from build123d import *

# Parameters (mm, degrees)
F0_W      = 114.3
F0_H      = 60.325
F1_DEPTH  = 42.8625
F2_W      = 98.425
F2_H      = 31.75
F3_DEPTH  = 25.4
F4_R      = 7.9375
F5_DEPTH  = 25.4
F10_DEPTH = 127


with BuildPart() as f1:
    # F0 (on Front) → F1 (new body, symmetric)
    with BuildSketch(Plane.XZ):
        with Locations((57.15, 30.1625)):
            Rectangle(F0_W, F0_H)
    extrude(amount=F1_DEPTH, both=True)

    # F2 (on face) → F3 (join)
    with BuildSketch(Plane.XY.offset(60.325)):
        with Locations((65.0875, -12.7)):
            Rectangle(F2_W, F2_H)
    extrude(amount=F3_DEPTH)

    # F4 (on face) → F5 (cut)
    with BuildSketch(Plane.XY.offset(60.325)):
        with Locations((31.8531343792, -12.7)):
            Circle(F4_R)
    extrude(amount=F5_DEPTH, mode=Mode.SUBTRACT)

    # F9 (on 3pt) → F10 (cut)
    with BuildSketch(Plane(origin=(85.5876450588, -49.4525301974, 49.4525301974), x_dir=(0.3874037681, 0.8943227315, 0.2238418469), z_dir=(0.7743554069, -0.4474224535, 0.4474224535))):
        Polygon((-14.9042876437, -25.4722796381), (7.5109787285, -51.4674633741), (114.2435371876, -48.7483553588), (131.361335516, 53.0414171517), (24.5024245232, 35.0616015494), (7.6925121248, 10.4205505922), align=None)
    extrude(amount=F10_DEPTH, mode=Mode.SUBTRACT)


solid = f1.part
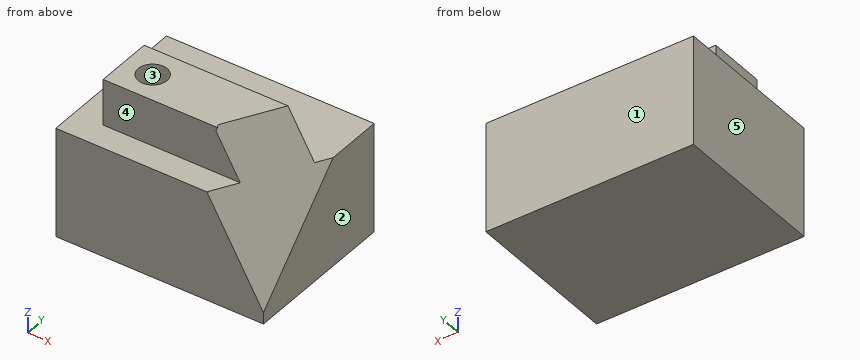
Work out the finished part from the listing and answer in its coordinate system (mm). Face numbers are marked on the shaded views. A direction names the side the tool comes from. Give positions to 0.01 mm unless a question says otherwise; leave off trailing zeros. Write each loop counter-clockwise with the first axis right and the second up, starting at its lowest first coordinate (ties: lowest second). Pieces come first, ordered by that corner, then holes. Notation, with made-up numbers: M 88.25,56 L 115.25,56 A19 ccw 115.25,70 Z; hole C 46,-23.75 d5. An arc over 180 degrees is marked long. Answer as CSV lines item,"result".
Q1. Given P1, Ø4, axis at x = 59.5, y = 14.5, coming from the +Z side (3 decimals); P2, Ø12.5, axis at x = 71.5, z = 74, coming from the -Y side (3 decimals); P3, Ø12.5, axis at x = 74, z = 68, coming from the +Y side (3 decimals), each flat-ended and moving along its own axis, determine where each tip first touches the part or whether it passes through.
A:
P1,"stops at z = 60.325"
P2,"stops at y = -28.575"
P3,"stops at y = 3.175"
Q2. A cutting plane is placed at C-C on z = 48. Write down the section's boundary in (x, y).
A:
outline,"M 0,-42.86 L 90.23,-42.86 L 114.3,-1.21 L 114.3,42.86 L 0,42.86 Z"
Q3. A tool of negligible diameter and unlimited length cuts with its end or side. For the marked faces 4 and 5, from which of +Z, -Z, +X, -X, +Y, -Y can it reach the whole face along a straight path? Write none if from no direction.
A:
face 4,"+Z, +X, -X, -Y"
face 5,"+Z, -Z, -X, +Y, -Y"
Q4. A cutting plane is placed at B-B on y = -1. Write down the section's boundary in (x, z) (1 decimal), plus the area to 3 significant figures.
A:
outline,"M 0,0 L 114.3,0 L 114.3,48.2 L 92.6,85.7 L 15.9,85.7 L 15.9,60.3 L 0,60.3 Z"
area,"8,990 mm²"
Q5. Find the intervals of material crossed by probe 1 along Z at (x, y) = (7.5, -11.5) (3 decimals); probe 2 along Y at (x, z) = (64.5, 66.5) (3 decimals); probe 3 along Y at (x, z) = (31, 63) (3 decimals), in increasing order. Write a range as [from, to].
A:
probe 1,"z = [0, 60.325]"
probe 2,"y = [-28.575, 3.175]"
probe 3,"y = [-28.575, -20.592], [-4.808, 3.175]"
Q6. A cutting plane is placed at D-D on y = -12.7. Write down the section's boundary in (x, z) (1 decimal).
A:
outline,"M 0,0 L 114.3,0 L 114.3,36.5 L 85.9,85.7 L 39.8,85.7 L 39.8,60.3 L 23.9,60.3 L 23.9,85.7 L 15.9,85.7 L 15.9,60.3 L 0,60.3 Z"
Q7. The mould has two halves that part along Y. Classify the marked faces 1, 2 and 3: +Y half, -Y half, draft (parallel to the pull), parting line (faces both ways), or undercut.
A:
face 1,"+Y half"
face 2,"draft"
face 3,"undercut"
Q8. A cutting plane is placed at A-A on x = 50. Write down the section's boundary in (y, z) (1 decimal).
A:
outline,"M -42.9,0 L 42.9,0 L 42.9,60.3 L 3.2,60.3 L 3.2,85.7 L -28.6,85.7 L -28.6,60.3 L -42.9,60.3 Z"
